Read the model definition and answer for the solid it produces. Units are mm, in the model's axes. Face numbers are marked on the shaded views. A direction names the side the tool comes from. Give positions to 0.01 mm unless a question says otherwise; leave off trailing zeros. Write each loop counter-clockwise with the first axis right and the second up, starting at its lowest first coordinate (ties: lowest second). Pieces come first, ordered by that corner, then holes. Notation, with made-up numbers: (-34, 33) -> (1, 33) arc R15 ccw to (1, 43) -> close; hole circle Ø6 at (58.25, 22.25). An arc over 180 degrees is marked (long way). Write item = value, one per line.
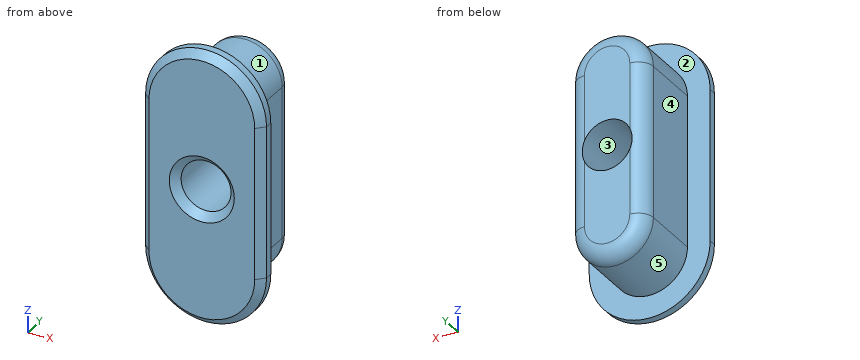
from build123d import *

# Parameters (mm, degrees)
PAD_DEPTH       = 2.5
PAD001_DEPTH    = 1
CHAMFER_SIZE    = 0.5
FILLET_R        = 1
SKETCH002_R     = 1.65
POCKET_DEPTH    = 6.001
CHAMFER001_SIZE = 0.5


with BuildPart() as part:
    # Sketch → Pad (new body, symmetric)
    with BuildSketch(Plane.XZ):
        with BuildLine():
            ThreePointArc((-2.5, -5), (0, -7.5), (2.5, -5))
            Line((2.5, -5), (2.5, 5))
            ThreePointArc((2.5, 5), (0, 7.5), (-2.5, 5))
            Line((-2.5, -5), (-2.5, 5))
        make_face()
    extrude(amount=PAD_DEPTH, both=True)

    # Sketch001 (on Face6 of Pad) → Pad001 (join)
    with BuildSketch(Plane.XZ.offset(2.5)):
        with BuildLine():
            ThreePointArc((4, 5), (0, 9), (-4, 5))
            Line((-4, 5), (-4, -5))
            ThreePointArc((-4, -5), (0, -9), (4, -5))
            Line((4, 5), (4, -5))
        make_face()
    extrude(amount=PAD001_DEPTH)

    # Chamfer
    chamfer_edges = [part.edges().sort_by_distance(p)[0] for p in [
        (0, -3.5, 9),
    ]]
    chamfer(chamfer_edges, length=CHAMFER_SIZE)

    # Fillet
    fillet_edges = [part.edges().sort_by_distance(p)[0] for p in [
        (0, 2.5, 7.5),
    ]]
    fillet(fillet_edges, radius=FILLET_R)

    # Sketch002 (on Face19 of Fillet) → Pocket (cut, through all)
    with BuildSketch(Plane.XZ.offset(3.5)):
        Circle(SKETCH002_R)
    extrude(amount=-POCKET_DEPTH, mode=Mode.SUBTRACT)

    # Chamfer001
    chamfer001_edges = [part.edges().sort_by_distance(p)[0] for p in [
        (-1.65, -3.5, 0),
    ]]
    chamfer(chamfer001_edges, length=CHAMFER001_SIZE)


solid = part.part
(1) Given P1, Ø3, axis at x = 2, y = 2, coming from the -Z side; P2, Ø1.2, axis at y = -1, z = 2, coming from the -X side; P3, Ø1, axis at y = -1, z = -4, coming from the +X side, each flat-ended and moving along its own axis, determine where each tip first touches the part or whether it passes through.
Checks:
P1 = -7.43
P2 = -2.5
P3 = 2.5
(2) The part is cut by section A-A on x = 0. Determine the outline of the cut face in (y, z), plus the area to 3 significant figures.
Checks:
outline = (-3.5, -8.5) -> (-3, -9) -> (-2.5, -9) -> (-2.5, -7.5) -> (1.5, -7.5) arc R1 ccw to (2.5, -6.5) -> (2.5, -1.65) -> (-3, -1.65) -> (-3.5, -2.15) -> close; (-3.5, 2.15) -> (-3, 1.65) -> (2.5, 1.65) -> (2.5, 6.5) arc R1 ccw to (1.5, 7.5) -> (-2.5, 7.5) -> (-2.5, 9) -> (-3, 9) -> (-3.5, 8.5) -> close
area = 72.3 mm²
(3) The part is cut by section B-B on z = 0. Determine the outline of the cut face in (x, y).
Checks:
outline = (-4, -3) -> (-3.5, -3.5) -> (-2.15, -3.5) -> (-1.65, -3) -> (-1.65, 2.49) arc R1 ccw to (-2.5, 1.5) -> (-2.5, -2.5) -> (-4, -2.5) -> close; (1.65, -3) -> (2.15, -3.5) -> (3.5, -3.5) -> (4, -3) -> (4, -2.5) -> (2.5, -2.5) -> (2.5, 1.5) arc R1 ccw to (1.65, 2.49) -> close
(4) Consider L1, parallel to X at y = -0.75, z = 0; L2, parallel to Z at x = 0, y = -0.1; L3, parallel to Y at x = 2.75, z = 0.5. Determine where each line is inside the solid, lowest interval first.
Checks:
L1 = -2.5 to -1.65, 1.65 to 2.5
L2 = -7.5 to -1.65, 1.65 to 7.5
L3 = -3.5 to -2.5
(5) The part is cut by section C-C on y = -1.5. Determine the outline of the cut face in (x, z), plus the area to 3 significant figures.
Checks:
outline = (-2.5, -5) arc R2.5 ccw to (2.5, -5) -> (2.5, 5) arc R2.5 ccw to (-2.5, 5) -> close; hole circle Ø3.3 at (0, 0)
area = 61.1 mm²
(6) A tool of negligible diameter and unlimited length cuts with its end or side. For the marked faces 1, 2, 3, 4 and 5, from which of +Z, -Z, +X, -X, +Y, -Y can it reach the whole face along a straight path? Write none if from no direction.
Checks:
face_1 = +Z, +Y
face_2 = +Y
face_3 = +Y, -Y
face_4 = +Z, -Z, -X, +Y
face_5 = -Z, +Y
